Here's how the part is built. I have some questions about the finished solid (model axes, mm). A direction names the side the tool comes from. Coordinates: 2 decimals unless noted, no trailing zeros. Order: outer loops, then holes, each group sorted by start corner. A loop starts at its lowest first (then second) coordinate and runs counter-clockwise, first axis right, second up. Notation, with made-up numbers: (6.5, 10.5) -> (38.5, 10.5) arc R7 cw to (38.5, 17.5) -> close; hole circle Ø1 at (7.5, 51.25). An arc over 180 degrees is marked (long way). One line per item, written item: value. Start each with the question number.
```python
from build123d import *

# Parameters (mm, degrees)
BOSS_EXTRUDE1_DEPTH = 35
SKETCH4_R           = 8
CUT_EXTRUDE1_DEPTH  = 112.130553854


with BuildPart() as part:
    # Sketch2 → Boss-Extrude1 (new, symmetric)
    with BuildSketch(Plane.XY):
        Polygon((-90, 0), (-40, 0), (-40, 40), (40, 40), (40, 0), (90, 0), (90, 15), (55, 15), (55, 55), (-55, 55), (-55, 15), (-90, 15), align=None)
    extrude(amount=BOSS_EXTRUDE1_DEPTH, both=True)

    # Sketch4 → Cut-Extrude1 (cut, through all)
    with BuildSketch(Plane(origin=(0, 55, 0), x_dir=(1, 0, 0), z_dir=(0, 1, 0))):
        with Locations(Location((0, 0, 0), (0, 0, 180))):
            Circle(SKETCH4_R)
        with BuildLine():
            Line((-70, 10), (-90, 10))
            Line((-90, 10), (-90, -10))
            Line((-90, -10), (-70, -10))
            ThreePointArc((-70, -10), (-60, 0), (-70, 10))
        make_face()
        with BuildLine():
            Line((90, -10), (90, 10))
            Line((90, 10), (70, 10))
            ThreePointArc((70, 10), (60, 0), (70, -10))
            Line((70, -10), (90, -10))
        make_face()
    extrude(amount=-CUT_EXTRUDE1_DEPTH, mode=Mode.SUBTRACT)

    # Sketch5 → Revolve1 (revolve)
    with BuildSketch(Plane.XY, mode=Mode.PRIVATE) as revolve1_sk:
        Polygon((-35, 105), (-20, 55), (-8, 55), (-8, 70), (-15, 85), (-15, 105), align=None)
    revolve(revolve1_sk.sketch.rotate(Axis((0, 55, 0), (0, 1, 0)), 180), axis=Axis((0, 55, 0), (0, 1, 0)))


solid = part.part
```
Q1. If we mould it in two halves opening along X, with no side actions, what happens to faces 1 (the face through (0.527, 55.21, -7.983)), 2 (the face through (55, 35, 0)), 3 (the face through (-5.577, 74.094, 25.117)), 4 (the face through (0, 44, 35))? For each: +X half, -X half, draft (parallel to the pull), parting line (faces both ways), or undercut.
Q2. Imagine slicing it at D-D (y = 98). Write out the boundary of the cut face in (x, z).
Q3. I need wall thicknesses on line 1 (X direction, y = 23, z = 22.5); line 2 (X direction, y = 6, z = -15); line 3 (Y direction, x = -80.5, z = -14.5). Which ranges of each line are inside material? Lowest first, please.
Q4. For faces 5 (the face through (8.06, 95.14, -12.65)), 6 (the face through (-80, 8, 10)), 7 (the face through (-40, 20, 0)), which set-ups out of +Z, -Z, +X, -X, +Y, -Y let a thin tool reach every point of the face, with its end or its side?
Q5. Imagine slicing it at C-C (x = 0). Write out the boundary of the cut face in (y, z).
Q6. For P1, Ø10, axis at y = 75, z = 0.5, coming from the -X side; P2, Ø3, axis at y = 66.5, z = 2, coming from the +X side; P3, Ø1.5, axis at y = 48.5, z = 2, coming from the +X side, each with a flat end and sliding along its axis, tell me the tip position at first contact or that it passes through.
Q7. Imagine slicing it at A-A (z = 0). Write out the boundary of the cut face in (x, y).
Q8. Imagine slicing it at B-B (y = 12.5). Write out the boundary of the cut face in (x, z), plus the area to 3 significant figures.
Completed:
1. face 1: undercut
1. face 2: +X half
1. face 3: parting line
1. face 4: draft
2. outline: circle Ø65.8 at (0, 0); hole circle Ø30 at (0, 0)
3. line 1: x = -55 to -40, 40 to 55
3. line 2: x = -90 to -40, 40 to 90
3. line 3: y = 0 to 15
4. face 5: +Y
4. face 6: -X, +Y, -Y
4. face 7: +Z, -Z, -Y
5. outline: (40, -35) -> (55, -35) -> (55, -20) -> (105, -35) -> (105, -15) -> (85, -15) -> (70, -8) -> (40, -8) -> close; (40, 8) -> (70, 8) -> (85, 15) -> (105, 15) -> (105, 35) -> (55, 20) -> (55, 35) -> (40, 35) -> close
6. P1: stops at x = -27.5
6. P2: stops at x = 23.83
6. P3: stops at x = 55
7. outline: (-60, 0) -> (-40, 0) -> (-40, 40) -> (-8, 40) -> (-8, 70) -> (-15, 85) -> (-15, 105) -> (-35, 105) -> (-20, 55) -> (-55, 55) -> (-55, 15) -> (-60, 15) -> close; (8, 40) -> (40, 40) -> (40, 0) -> (60, 0) -> (60, 15) -> (55, 15) -> (55, 55) -> (20, 55) -> (35, 105) -> (15, 105) -> (15, 85) -> (8, 70) -> close
8. outline: (-90, -35) -> (-40, -35) -> (-40, 35) -> (-90, 35) -> (-90, 10) -> (-70, 10) arc R10 cw to (-70, -10) -> (-90, -10) -> close; (40, -35) -> (90, -35) -> (90, -10) -> (70, -10) arc R10 cw to (70, 10) -> (90, 10) -> (90, 35) -> (40, 35) -> close
8. area: 5,890 mm2
